The listing builds one solid part. Answer for the finished solid, in the listing's coordinates (mm). Round coordinates to 2 decimals unless told otherwise and drop trailing zeros. Order: outer loops, then holes, each group sorted by start corner. A loop starts at its lowest first (then second) coordinate and runs counter-clockwise, first axis right, second up. Notation, with made-up numbers: M -10.5,-2.5 L 17.5,-2.5 A22 cw 17.5,24.5 Z; hole C -7.5,2.25 d5. An arc over 180 degrees is marked long. Put each result on its own line as item: value. Start each with the question number.
1. Each of these flat-tipped pins is pushed along its axis until it touches: pin 1 Ø2 at (x, y) = (97, -4) entering from -Z; pin 2 Ø2.5 at (x, y) = (18, -2.5) entering from +Z; pin 3 Ø3 at (y, z) = (-3, -90) entering from +X. Where does it stop, or does it pass through?
2. The part is cut by section A-A (z = 36). Give the vertices of the cut face in (x, y).
3. The part is cut by section D-D (y = -1.7). Count the separate pieces of the cut face and the enclosed holes in it, then the cut area to 3 significant figures.
4. The part is cut by section C-C (z = -115). Give the vertices of the cut face in (x, y).
5. Consider line 1 (Z direction, x = -89, y = -2.1); line 2 (X direction, y = -3, z = -45.5); line 3 (Z direction, x = -40.5, y = -3.05). Determine where each line is inside the solid, lowest interval first.
6. The part is cut by section B-B (x = -115). Give the vertices of the cut face in (y, z), then the cut area to 3 significant figures.
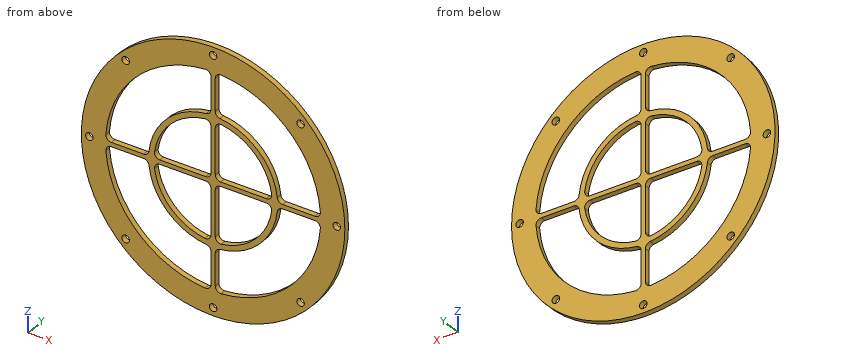
from build123d import *

# Parameters (mm, degrees)
F0_R     = 122.5
F0_R_2   = 3.5
F1_DEPTH = 5


# Not quite as in the source:
# - a feature names something its author has since deleted; it is built from what else it names


with BuildPart() as f1:
    # F0 (on Front) → F1 (new body)
    with BuildSketch(Plane.XZ):
        Circle(F0_R)
        with Locations((-81.3172798365, -81.3172798365)):
            Circle(F0_R_2, mode=Mode.SUBTRACT)
        with BuildLine():
            ThreePointArc((-99.7281623775, -7.3684210526), (-98.4052297439, -3.5972147631), (-94.7417542586, -2))
            Line((-94.7417542586, -2), (-64.6219776856, -2))
            ThreePointArc((-64.6219776856, -2), (-61.2822402478, -3.2789579623), (-59.6510563252, -6.4615384615))
            ThreePointArc((-59.6510563252, -6.4615384615), (-42.4264068712, -42.4264068712), (-6.4615384615, -59.6510563252))
            ThreePointArc((-6.4615384615, -59.6510563252), (-3.2789579623, -61.2822402478), (-2, -64.6219776856))
            Line((-2, -64.6219776856), (-2, -94.7417542586))
            ThreePointArc((-2, -94.7417542586), (-3.5972147631, -98.4052297439), (-7.3684210526, -99.7281623775))
            ThreePointArc((-7.3684210526, -99.7281623775), (-70.7106781187, -70.7106781187), (-99.7281623775, -7.3684210526))
        make_face(mode=Mode.SUBTRACT)
        with BuildLine():
            ThreePointArc((-7, -2), (-3.4644660941, -3.4644660941), (-2, -7))
            Line((-2, -7), (-2, -49.5075751779))
            ThreePointArc((-2, -49.5075751779), (-3.7212807378, -53.2824923956), (-7.7, -54.4583326957))
            ThreePointArc((-7.7, -54.4583326957), (-38.8908729653, -38.8908729653), (-54.4583326957, -7.7))
            ThreePointArc((-54.4583326957, -7.7), (-53.2824923956, -3.7212807378), (-49.5075751779, -2))
            Line((-49.5075751779, -2), (-7, -2))
        make_face(mode=Mode.SUBTRACT)
        with Locations((0, -115)):
            Circle(F0_R_2, mode=Mode.SUBTRACT)
        with Locations((81.3172798365, -81.3172798365)):
            Circle(F0_R_2, mode=Mode.SUBTRACT)
        with BuildLine():
            ThreePointArc((99.7281623775, -7.3684210526), (70.7106781187, -70.7106781187), (7.3684210526, -99.7281623775))
            ThreePointArc((7.3684210526, -99.7281623775), (3.5972147631, -98.4052297439), (2, -94.7417542586))
            Line((2, -94.7417542586), (2, -64.6219776856))
            ThreePointArc((2, -64.6219776856), (3.2789579623, -61.2822402478), (6.4615384615, -59.6510563252))
            ThreePointArc((6.4615384615, -59.6510563252), (42.4264068712, -42.4264068712), (59.6510563252, -6.4615384615))
            ThreePointArc((59.6510563252, -6.4615384615), (61.2822402478, -3.2789579623), (64.6219776856, -2))
            Line((64.6219776856, -2), (94.7417542586, -2))
            ThreePointArc((94.7417542586, -2), (98.4052297439, -3.5972147631), (99.7281623775, -7.3684210526))
        make_face(mode=Mode.SUBTRACT)
        with BuildLine():
            Line((2, -49.5075751779), (2, -7))
            ThreePointArc((2, -7), (3.4644660941, -3.4644660941), (7, -2))
            Line((7, -2), (49.5075751779, -2))
            ThreePointArc((49.5075751779, -2), (53.2824923956, -3.7212807378), (54.4583326957, -7.7))
            ThreePointArc((54.4583326957, -7.7), (38.8908729653, -38.8908729653), (7.7, -54.4583326957))
            ThreePointArc((7.7, -54.4583326957), (3.7212807378, -53.2824923956), (2, -49.5075751779))
        make_face(mode=Mode.SUBTRACT)
        with Locations((-115, 0)):
            Circle(F0_R_2, mode=Mode.SUBTRACT)
        with BuildLine():
            ThreePointArc((-2, 7), (-3.4644660941, 3.4644660941), (-7, 2))
            Line((-7, 2), (-49.5075751779, 2))
            ThreePointArc((-49.5075751779, 2), (-53.2824923956, 3.7212807378), (-54.4583326957, 7.7))
            ThreePointArc((-54.4583326957, 7.7), (-38.8908729653, 38.8908729653), (-7.7, 54.4583326957))
            ThreePointArc((-7.7, 54.4583326957), (-3.7212807378, 53.2824923956), (-2, 49.5075751779))
            Line((-2, 49.5075751779), (-2, 7))
        make_face(mode=Mode.SUBTRACT)
        with BuildLine():
            ThreePointArc((-99.7281623775, 7.3684210526), (-70.7106781187, 70.7106781187), (-7.3684210526, 99.7281623775))
            ThreePointArc((-7.3684210526, 99.7281623775), (-3.5972147631, 98.4052297439), (-2, 94.7417542586))
            Line((-2, 94.7417542586), (-2, 64.6219776856))
            ThreePointArc((-2, 64.6219776856), (-3.2789579623, 61.2822402478), (-6.4615384615, 59.6510563252))
            ThreePointArc((-6.4615384615, 59.6510563252), (-42.4264068712, 42.4264068712), (-59.6510563252, 6.4615384615))
            ThreePointArc((-59.6510563252, 6.4615384615), (-61.2822402478, 3.2789579623), (-64.6219776856, 2))
            Line((-64.6219776856, 2), (-94.7417542586, 2))
            ThreePointArc((-94.7417542586, 2), (-98.4052297439, 3.5972147631), (-99.7281623775, 7.3684210526))
        make_face(mode=Mode.SUBTRACT)
        with Locations((-81.3172798365, 81.3172798365)):
            Circle(F0_R_2, mode=Mode.SUBTRACT)
        with BuildLine():
            Line((49.5075751779, 2), (7, 2))
            ThreePointArc((7, 2), (3.4644660941, 3.4644660941), (2, 7))
            Line((2, 7), (2, 49.5075751779))
            ThreePointArc((2, 49.5075751779), (3.7212807378, 53.2824923956), (7.7, 54.4583326957))
            ThreePointArc((7.7, 54.4583326957), (38.8908729653, 38.8908729653), (54.4583326957, 7.7))
            ThreePointArc((54.4583326957, 7.7), (53.2824923956, 3.7212807378), (49.5075751779, 2))
        make_face(mode=Mode.SUBTRACT)
        with BuildLine():
            Line((2, 64.6219776856), (2, 94.7417542586))
            ThreePointArc((2, 94.7417542586), (3.5972147631, 98.4052297439), (7.3684210526, 99.7281623775))
            ThreePointArc((7.3684210526, 99.7281623775), (70.7106781187, 70.7106781187), (99.7281623775, 7.3684210526))
            ThreePointArc((99.7281623775, 7.3684210526), (98.4052297439, 3.5972147631), (94.7417542586, 2))
            Line((94.7417542586, 2), (64.6219776856, 2))
            ThreePointArc((64.6219776856, 2), (61.2822402478, 3.2789579623), (59.6510563252, 6.4615384615))
            ThreePointArc((59.6510563252, 6.4615384615), (42.4264068712, 42.4264068712), (6.4615384615, 59.6510563252))
            ThreePointArc((6.4615384615, 59.6510563252), (3.2789579623, 61.2822402478), (2, 64.6219776856))
        make_face(mode=Mode.SUBTRACT)
        with Locations((115, 0)):
            Circle(F0_R_2, mode=Mode.SUBTRACT)
        with Locations((0, 115)):
            Circle(F0_R_2, mode=Mode.SUBTRACT)
        with Locations((81.3172798365, 81.3172798365)):
            Circle(F0_R_2, mode=Mode.SUBTRACT)
    extrude(amount=F1_DEPTH)


solid = f1.part
Resolved:
1. pin 1: z = -76.09
1. pin 2: z = 121.35
1. pin 3: x = 84.7
2. outline: M -117.09,-5 L -93.3,-5 L -93.3,0 L -117.09,0 Z; M -48,-5 L -41.58,-5 L -41.58,0 L -48,0 Z; M -2,-5 L 2,-5 L 2,0 L -2,0 Z; M 41.58,-5 L 48,-5 L 48,0 L 41.58,0 Z; M 93.3,-5 L 117.09,-5 L 117.09,0 L 93.3,0 Z
3. separate pieces: 1
3. enclosed holes: 16
3. area: 18,900 mm2
4. outline: M -42.2,-5 L -3.5,-5 L -3.5,0 L -42.2,0 Z; M 3.5,-5 L 42.2,-5 L 42.2,0 L 3.5,0 Z
5. line 1: -84.17 to -45.6, -2 to 2, 45.6 to 84.17
5. line 2: -113.74 to -89.05, -39.11 to -30.9, -2 to 2, 30.9 to 39.11, 89.05 to 113.74
5. line 3: -115.61 to -91.43, -44.27 to -37.21, -2 to 2, 37.21 to 44.27, 91.43 to 115.61
6. outline: M -5,-42.2 L 0,-42.2 L 0,-3.5 L -5,-3.5 Z; M -5,3.5 L 0,3.5 L 0,42.2 L -5,42.2 Z
6. area: 387 mm2
